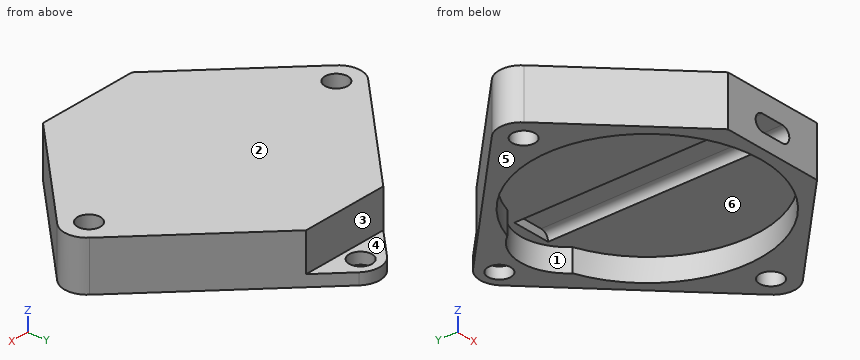
```python
from build123d import *

# Parameters (mm, degrees)
BOSS_EXTRUDE1_DEPTH = 4.35
SKETCH1_3_R         = 1
CUT_EXTRUDE1_DEPTH  = 5.35
SKETCH1_4_R         = 10
SKETCH1_4_R_2       = 4.1
CUT_EXTRUDE2_DEPTH  = 2
FILLET1_R           = 2
CUT_EXTRUDE3_DEPTH  = 5.35
CUT_EXTRUDE4_DEPTH  = 21.2
CUT_EXTRUDE5_DEPTH  = 3.35


with BuildPart() as part:
    # Sketch1 → Boss-Extrude1 (new body)
    with BuildSketch(Plane.XY):
        Polygon((0, 15.5), (-15.5, 0), (0, -15.5), (15.5, 0), align=None)
    extrude(amount=BOSS_EXTRUDE1_DEPTH)

    # Sketch1<3> → Cut-Extrude1 (cut, through all)
    with BuildSketch(Plane.XY):
        with Locations((-12.5, 0)):
            Circle(SKETCH1_3_R)
        with Locations((12.5, 0)):
            Circle(SKETCH1_3_R)
        with Locations((0, 13)):
            Circle(SKETCH1_3_R)
    extrude(amount=CUT_EXTRUDE1_DEPTH, mode=Mode.SUBTRACT)

    # Sketch1<4> → Cut-Extrude2 (cut)
    with BuildSketch(Plane.XY):
        Circle(SKETCH1_4_R)
        with Locations((0, 7)):
            Circle(SKETCH1_4_R_2)
    extrude(amount=CUT_EXTRUDE2_DEPTH, mode=Mode.SUBTRACT)

    # Fillet1
    fillet1_edges = [part.edges().sort_by_distance(p)[0] for p in [
        (0, -15.5, 2.175),
        (-15.5, 0, 2.175),
        (0, 15.5, 2.175),
        (15.5, 0, 2.175),
    ]]
    fillet(fillet1_edges, radius=FILLET1_R)

    # Sketch2 → Cut-Extrude3 (cut, through all)
    with BuildSketch(Plane(origin=(0, 0, 0), x_dir=(-1, 0, 0), z_dir=(0, 0, -1))):
        with BuildLine():
            Line((4.5, -11), (-4.5, -11))
            Line((-4.5, -11), (-1.414213562, -14.085786438))
            ThreePointArc((-1.414213562, -14.085786438), (0, -14.671572875), (1.414213562, -14.085786438))
            Line((1.414213562, -14.085786438), (4.5, -11))
        make_face()
    extrude(amount=-CUT_EXTRUDE3_DEPTH, mode=Mode.SUBTRACT)

    # Sketch4 → Cut-Extrude4 (cut)
    with BuildSketch(Plane.XZ.offset(11)):
        with BuildLine():
            Line((-1, 2.7), (1, 2.7))
            ThreePointArc((1, 2.7), (1.7, 2), (1, 1.3))
            Line((1, 1.3), (-1, 1.3))
            ThreePointArc((-1, 1.3), (-1.7, 2), (-1, 2.7))
        make_face()
    extrude(amount=-CUT_EXTRUDE4_DEPTH, mode=Mode.SUBTRACT)

    # Sketch11 → Cut-Extrude5 (cut)
    with BuildSketch(Plane.XY.offset(4.35)):
        Polygon((-3.9, 11.6), (3.9, 11.6), (0, 15.5), align=None)
    extrude(amount=-CUT_EXTRUDE5_DEPTH, mode=Mode.SUBTRACT)


solid = part.part
```
Verification items for the finished model (mm, model axes). Face numbers are marked on the shaded views. A direction names the side the tool comes from. Round coordinates to 2 decimals unless told otherwise and drop trailing zeros. Loops run counter-clockwise (first coordinate to the right, second up) from the corner with the lowest first, then second, coordinate; pieces in that order, holes last. Notation, with made-up numbers: (75.5, -26.75) -> (101.5, -26.75) arc R16 ccw to (101.5, -11.75) -> close; hole circle Ø1 at (-7.5, 3). An arc over 180 degrees is marked (long way). Answer as a JSON object with one key per item and string values.
Q1. Draft check along Y on the marked faces 1, 2 and 3. Enter one of: pulls with the +Y half, pulls with the -Y half, needs draft (parallel to the pull), parting line crosses it, or undercut.
Data:
{"face 1": "undercut", "face 2": "needs draft", "face 3": "pulls with the +Y half"}
Q2. Section check A-A (y = 0). Record the boundary of the cut face in (x, z).
Data:
{"outline": "(-14.67, 0) -> (-13.5, 0) -> (-13.5, 4.35) -> (-14.67, 4.35) -> close; (-11.5, 0) -> (-10, 0) -> (-10, 2) -> (-1.7, 2) arc R0.7 cw to (-1, 2.7) -> (1, 2.7) arc R0.7 cw to (1.7, 2) -> (10, 2) -> (10, 0) -> (11.5, 0) -> (11.5, 4.35) -> (-11.5, 4.35) -> close; (13.5, 0) -> (14.67, 0) -> (14.67, 4.35) -> (13.5, 4.35) -> close"}
Q3. Section check C-C (y = 13). Record the boundary of the cut face in (x, z), then the cut area to 3 significant figures.
Data:
{"outline": "(-2.5, 0) -> (-1, 0) -> (-1, 1) -> (-2.5, 1) -> close; (1, 0) -> (2.5, 0) -> (2.5, 1) -> (1, 1) -> close", "area": "3.00 mm2"}
Q4. Section check D-D (y = -4.5). Record the boundary of the cut face in (x, z).
Data:
{"outline": "(-11, 0) -> (-8.93, 0) -> (-8.93, 2) -> (-1.7, 2) arc R0.7 cw to (-1, 2.7) -> (1, 2.7) arc R0.7 cw to (1.7, 2) -> (8.93, 2) -> (8.93, 0) -> (11, 0) -> (11, 4.35) -> (-11, 4.35) -> close"}
Q5. Go/stop test with flat-tipped pins: P1, Ø12, axis at x = 0, y = 0, coming from the -Z side; P2, Ø2, axis at x = -0.5, y = -5, coming from the -Z side; P3, Ø1.7, axis at x = -1.5, z = 2, coming from the +Y side. Record where each tip stops, or that it passes through.
Data:
{"P1": "stops at z = 2", "P2": "stops at z = 2.49", "P3": "stops at y = 11.6"}
Q6. Access from +Z, -Z, +X, -X, +Y, -Y to the whole of each face (thin tool, end or side, straight path). Record for the marked faces 4, 5 and 6.
Data:
{"face 4": "+Z, +X, -X, +Y", "face 5": "-Z, +X, -X, +Y, -Y", "face 6": "-Z"}
Q7. Section check B-B (x = 12.5). Record the boundary of the cut face in (y, z).
Data:
{"outline": "(-3, 0) -> (-1, 0) -> (-1, 4.35) -> (-3, 4.35) -> close; (1, 0) -> (3, 0) -> (3, 4.35) -> (1, 4.35) -> close"}
Q8. Scan lines: line 1 (Y direction, x = 0, z = 0.4); line 2 (X direction, y = 0, z = 1.1); line 3 (Y direction, x = 0, z = 3.35). Record each from-to range of solid material in increasing order. Write a range as from..to.
Data:
{"line 1": "y = -11..-10, 11.1..12, 14..14.67", "line 2": "x = -14.67..-13.5, -11.5..-10, 10..11.5, 13.5..14.67", "line 3": "y = -11..11.6"}
